Build history of the part. All positions in model axes, mm. Give positions to 0.01 mm unless a question says otherwise; leave off trailing zeros. Write each loop counter-clockwise with the first axis right and the second up, starting at its lowest first coordinate (ties: lowest second). Pieces come first, ordered by that corner, then holes.
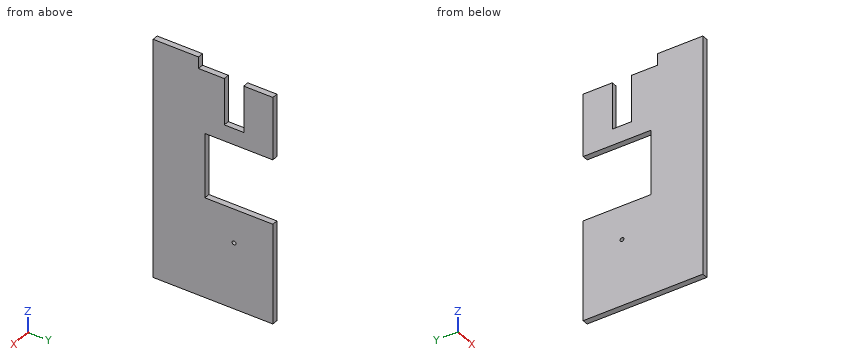
from build123d import *

# Parameters (mm, degrees)
F0_R     = 6
F1_DEPTH = 18


with BuildPart() as f1:
    # F0 (on Right) → F1 (new body)
    with BuildSketch(Plane.YZ):
        Polygon((0, 740), (0, 0), (370, 0), (370, 310), (160, 310), (160, 510), (370, 510), (370, 704), (280, 704), (280, 560), (220, 560), (220, 704), (140, 704), (140, 740), align=None)
        with Locations((250, 205)):
            Circle(F0_R, mode=Mode.SUBTRACT)
    extrude(amount=F1_DEPTH)


solid = f1.part
1. Saw through at B-B on z = 626. Give the cut face in (x, y).
2. Drop flat-ended pins along their axis: pin 1 (9 mm diameter, centred on x = 7.5, y = 263.5, fed in from +Z); pin 2 (7 mm diameter, centred on y = 250, z = 205, fed in from -X). Give the stop position or say it passes through.
3. Drill centre lines: line 1 along Z through (x, y) = (5.75, 250); line 2 along Z through (x, y) = (16.25, 227); line 3 along Y through (x, z) = (8.25, 638). Where is each one in solid material? Low to high.
4. Saw through at C-C on x = 7.5. Give the cut face in (y, z).
5. Saw through at A-A on y = 227. Give the cut face in (x, z), plus the area to 3 significant figures.
6. Saw through at D-D on z = 468.5. Give the cut face in (x, y), plus the area to 3 significant figures.
Outcome:
1. outline: (0, 0) - (18, 0) - (18, 220) - (0, 220) - close; (0, 280) - (18, 280) - (18, 370) - (0, 370) - close
2. pin 1: stops at z = 560
2. pin 2: passes through
3. line 1: z = 0 to 199, 211 to 310, 510 to 560
3. line 2: z = 0 to 310, 510 to 560
3. line 3: y = 0 to 220, 280 to 370
4. outline: (0, 0) - (370, 0) - (370, 310) - (160, 310) - (160, 510) - (370, 510) - (370, 704) - (280, 704) - (280, 560) - (220, 560) - (220, 704) - (140, 704) - (140, 740) - (0, 740) - close; hole circle Ø12 at (250, 205)
5. outline: (0, 0) - (18, 0) - (18, 310) - (0, 310) - close; (0, 510) - (18, 510) - (18, 560) - (0, 560) - close
5. area: 6,480 mm2
6. outline: (0, 0) - (18, 0) - (18, 160) - (0, 160) - close
6. area: 2,880 mm2
